Model file for the job. Use its own axes, mm. A direction names the side the tool comes from. Give positions to 0.01 mm unless a question says otherwise; leave off trailing zeros. Write each loop counter-clockwise with the first axis right and the second up, starting at its lowest first coordinate (ties: lowest second). Pieces come first, ordered by that corner, then holes. Notation, with made-up numbers: (-29.75, 53.25) - (6.25, 53.25) arc R10 ccw to (6.25, 58.25) - close; hole circle Ø5 at (23, 12.5). An arc over 180 degrees is marked (long way). One line per item, written item: value. Start each with the question number.
(1) Cut at C-C, the plane y = -5.5. List the corners of the cut face in (x, z) (3 decimals), and give its area (3 significant figures).
(2) 3-axis set-ups, long thin cutter, end or side, ignore diameter. For faces 1 (the face through (28.68, -5.91, 11.66)), 2 (the face through (19.267, -18.044, 13.361)), 3 (the face through (25.4, -29, 21)), 4 (the face through (28, -19, 28.575)): which of +Z, -Z, +X, -X, +Y, -Y reach the whole face in a straight line?
(3) Cut at B-B, the plane x = 24. List the corners of the cut face in (y, z) (3 decimals).
(4) Probe L1, parallel to Y at x = 30.5, z = 19.5; L2, parallel to Y at x = 3.5, z = 15; L3, parallel to X at y = -20, z = 18. List the from-to ranges inside material, lowest first.
(5) Cut at A-A, the plane z = 7. List the corners of the cut face in (x, y).
(6) Drop flat-ended pins along their axis: P1, Ø4, axis at y = -18.5, z = 15, coming from the -X side; P2, Ø1.7, axis at y = -24, z = 23, coming from the -X side; P3, Ø4, axis at x = 11.5, y = -19, coming from the +Z side (3 decimals). Give the stop position or say it passes through.
(7) Mould opens along Y. For faces 5 (the face through (22.2, -4.7, 30.1)), 6 (the face through (27.996, -6.994, 35.296)), 7 (the face through (19.32, -3.13, 19.32)) say: pulls with the +Y half, pulls with the -Y half, needs draft (parallel to the pull), parting line crosses it, or undercut.
(8) Cut at D-D, the plane x = 9.5. List the corners of the cut face in (y, z) (3 decimals).
from build123d import *

# Parameters (mm, degrees)
F0_W      = 38.1
F0_H      = 38.1
F1_DEPTH  = 38.1
F6_DEPTH  = 38.1
F8_DEPTH  = 38.1
F9_W      = 25.4
F9_H      = 7.62
F10_DEPTH = 38.1


with BuildPart() as f1:
    # F0 (on Front) → F1 (new body)
    with BuildSketch(Plane.XZ):
        with Locations((19.05, 19.05)):
            Rectangle(F0_W, F0_H)
    extrude(amount=F1_DEPTH)

    # F5 (on offset) → F6 (cut)
    with BuildSketch(Plane.YZ.offset(38.1)):
        Polygon((-11.400602, 16.104914), (-6.35, 38.1), (-31.75, 38.1), (-26.640602, 16.104914), (-21.560602, 28.575), (-16.480602, 28.575), align=None)
        Polygon((-6.35, 0), (0, 0), (0, 38.1), align=None)
        Polygon((-25.4, 0), (-12.7, 0), (-19.05, 15.875), align=None)
        Polygon((-38.1, 0), (-31.75, 0), (-38.1, 38.1), align=None)
    extrude(amount=-F6_DEPTH, mode=Mode.SUBTRACT)

    # F7 (on offset) → F8 (cut)
    with BuildSketch(Plane.XZ.offset(38.1)):
        Polygon((0, 38.1), (0, 0), (6.35, 38.1), align=None)
        Polygon((25.4, 38.1), (12.7, 38.1), (19.05, 22.225), align=None)
        Polygon((31.75, 38.1), (38.1, 0), (38.1, 38.1), align=None)
        Polygon((11.43, 20.184822), (6.35, 0), (31.75, 0), (26.67, 19.299196), (21.59, 9.525), (16.51, 9.525), align=None)
    extrude(amount=-F8_DEPTH, mode=Mode.SUBTRACT)

    # F9 (on offset) → F10 (cut)
    with BuildSketch(Plane.XY.offset(38.1)):
        with Locations((12.7, -26.67)):
            Rectangle(F9_W, F9_H)
        with Locations((25.4, -11.43)):
            Rectangle(F9_W, F9_H)
    extrude(amount=-F10_DEPTH, mode=Mode.SUBTRACT)


solid = f1.part
Answers follow:
1. outline: (0.85, 5.1) - (7.634, 5.1) - (11.43, 20.185) - (16.51, 9.525) - (21.59, 9.525) - (26.67, 19.299) - (30.408, 5.1) - (37.25, 5.1) - (31.75, 38.1) - (25.4, 38.1) - (19.05, 22.225) - (12.7, 38.1) - (6.35, 38.1) - close
1. area: 744 mm²
2. face 1: -Z, +Y, -Y
2. face 2: -Z, +X, -X
2. face 3: +Z, -Z, -X
2. face 4: +Z, +X, -X
3. outline: (-37.517, 34.6) - (-34.11, 14.162) - (-30.48, 14.162) - (-30.48, 32.633) - (-30.937, 34.6) - close; (-22.86, 14.162) - (-19.735, 14.162) - (-19.05, 15.875) - (-18.365, 14.162) - (-15.24, 14.162) - (-15.24, 25.53) - (-16.481, 28.575) - (-21.561, 28.575) - (-22.86, 25.385) - close; (-7.62, 14.162) - (-3.99, 14.162) - (-0.583, 34.6) - (-7.154, 34.6) - (-7.62, 32.569) - close
4. L1: y = -35 to -27.43, -25.26 to -15.24, -7.62 to -3.1
4. L2: y = -34.25 to -30.48, -22.86 to -19.4, -18.7 to -3.85
4. L3: x = 3 to 10.88, 12.47 to 25.99, 27.01 to 35.1
5. outline: (1.17, -32.92) - (8.11, -32.92) - (8.11, -30.48) - (1.17, -30.48) - close; (1.17, -22.86) - (8.11, -22.86) - (8.11, -22.6) - (1.17, -22.6) - close; (1.17, -15.5) - (8.11, -15.5) - (8.11, -5.18) - (1.17, -5.18) - close; (29.91, -32.92) - (36.93, -32.92) - (36.93, -22.6) - (29.91, -22.6) - close; (29.91, -15.5) - (36.93, -15.5) - (36.93, -15.24) - (29.91, -15.24) - close; (29.91, -7.62) - (36.93, -7.62) - (36.93, -5.18) - (29.91, -5.18) - close
6. P1: stops at x = 2.18
6. P2: stops at x = 25.4
6. P3: stops at z = 28.575
7. face 5: needs draft
7. face 6: undercut
7. face 7: pulls with the +Y half
8. outline: (-38.1, 38.1) - (-33.836, 12.516) - (-30.48, 12.516) - (-30.48, 32.633) - (-31.75, 38.1) - close; (-22.86, 12.516) - (-20.394, 12.516) - (-19.05, 15.875) - (-17.706, 12.516) - (-4.264, 12.516) - (0, 38.1) - (-6.35, 38.1) - (-11.401, 16.105) - (-16.481, 28.575) - (-21.561, 28.575) - (-22.86, 25.385) - close
